Geometry: see drawing. Coordinates: mm, zero at the bounding-box minimum. A direction names the side the tool comes from. Give positions to 0.01 mm unless a question says otherwise; leave off trailing zeros. Order: outer loops, then holes, each group sorted by start corner. A loop starts at its lowest first (then second) coordinate and runs counter-clockwise, first axis right, second up. Notation, with made-up numbers: (-5.5, 51) - (18.5, 51) arc R10 ccw to (18.5, 70) - close; hole circle Ø8 at (15.25, 67). An arc over 180 degrees is marked (long way). Write each question's results on one line, items separated by ' | '. Start each with the question number.
Item 1: Mould query, pull axis X, two halves, no side actions, for the marked faces 1, 2 and 3. Classes: released by +X, released by -X, zero draft, split by the parting line, or undercut.
Item 2: Line query: line 1 along Z through (x, y) = (10, 11.25); line 2 along X through (y, z) = (0.75, 8.75); line 3 along X through (y, z) = (9.75, 5). Output: solid intervals per line, ascending.
Item 3: Section D-D on z = 8.5. Output: boundary loops of the cut face in (x, y), and give its area (4 significant figures).
Item 4: Contact query for a flat-ended pin moving along its axis: pin 1 Ø4 at (x, z) = (10, 5) entering from -Y. Output: stop coordinate, or through.
Item 5: Section B-B on y = 3.5. Output: boundary loops of the cut face in (x, z), and give its area (3 significant figures).
Item 6: Set-up query: the marked faces 4 and 5. Return all of +Z, -Z, +X, -X, +Y, -Y with unobstructed straight access to the full face (end or side cutting, diameter ignored); none if empty.
Item 7: Section A-A on x = 10. Output: boundary loops of the cut face in (y, z).
Item 8: Section C-C on z = 6.25. Output: boundary loops of the cut face in (x, y), and give its area (3 significant figures).
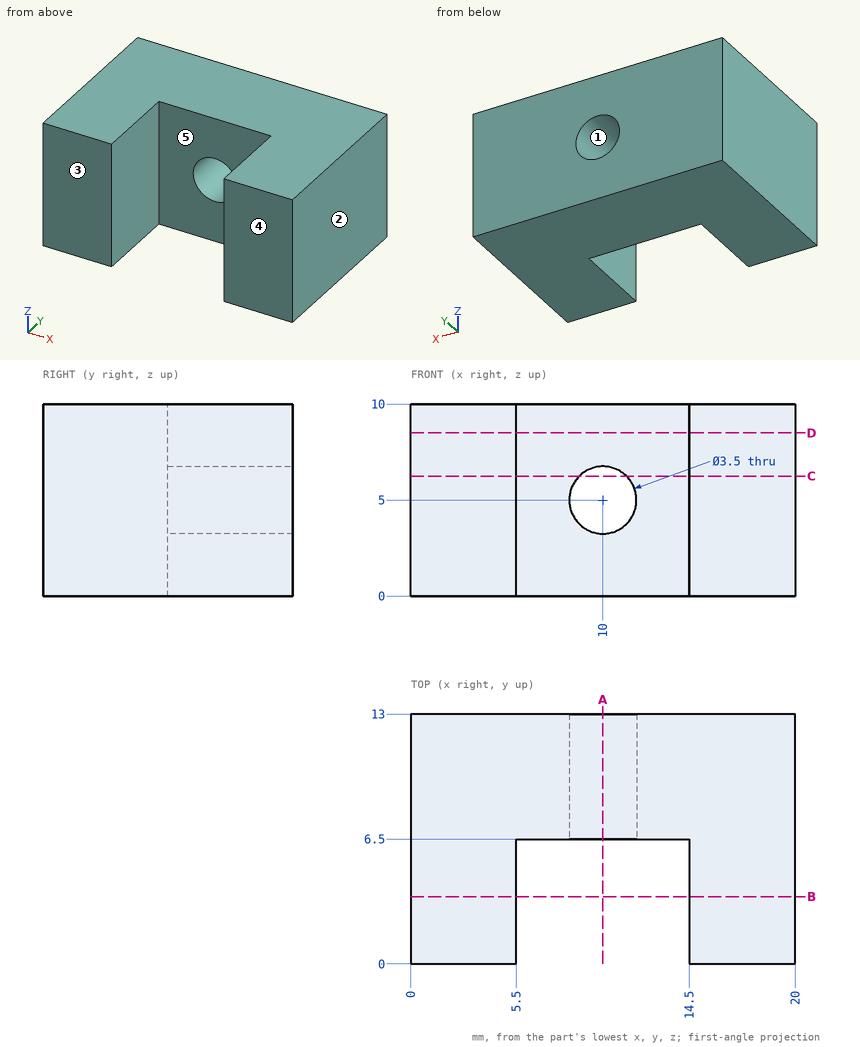
Evaluation:
1) face 1: undercut | face 2: released by +X | face 3: zero draft
2) line 1: z = 0 to 3.25, 6.75 to 10 | line 2: x = 0 to 5.5, 14.5 to 20 | line 3: x = 0 to 8.25, 11.75 to 20
3) outline: (0, 0) - (5.5, 0) - (5.5, 6.5) - (14.5, 6.5) - (14.5, 0) - (20, 0) - (20, 13) - (0, 13) - close | area: 201.5 mm^2
4) pin 1: stops at y = 6.5
5) outline: (0, 0) - (5.5, 0) - (5.5, 10) - (0, 10) - close; (14.5, 0) - (20, 0) - (20, 10) - (14.5, 10) - close | area: 110 mm^2
6) face 4: +Z, -Z, +X, -X, -Y | face 5: +Z, -Z, -Y
7) outline: (6.5, 0) - (13, 0) - (13, 3.25) - (6.5, 3.25) - close; (6.5, 6.75) - (13, 6.75) - (13, 10) - (6.5, 10) - close
8) outline: (0, 0) - (5.5, 0) - (5.5, 6.5) - (8.78, 6.5) - (8.78, 13) - (0, 13) - close; (11.22, 6.5) - (14.5, 6.5) - (14.5, 0) - (20, 0) - (20, 13) - (11.22, 13) - close | area: 186 mm^2
